from build123d import *

# Parameters (mm, degrees)
SKETCH1_W           = 24
SKETCH1_H           = 6
SKETCH1_H_2         = 24
SKETCH1_W_2         = 6
SKETCH1_R           = 1.625
BOSS_EXTRUDE1_DEPTH = 1.6
FILLET1_R           = 3.5
FILLET2_R           = 5


with BuildPart() as part:
    # Sketch1 → Boss-Extrude1 (new body)
    # profile 1 of 7: a face of its own
    with BuildSketch(Plane(origin=(0, 0, 0), x_dir=(1, 0, 0), z_dir=(0, 1, 0))):
        with Locations((0, 15)):
            Rectangle(SKETCH1_W, SKETCH1_H)
    # profile 2 of 7: a face of its own
    with BuildSketch(Plane(origin=(0, 0, 0), x_dir=(1, 0, 0), z_dir=(0, 1, 0))):
        Rectangle(SKETCH1_W, SKETCH1_H_2)
    # profile 3 of 7: a face of its own
    with BuildSketch(Plane(origin=(0, 0, 0), x_dir=(1, 0, 0), z_dir=(0, 1, 0))):
        with Locations((15, -15)):
            Rectangle(SKETCH1_W_2, SKETCH1_H)
        with Locations(Location((15.25, -15.25, 0), (0, 0, 270))):
            Circle(SKETCH1_R, mode=Mode.SUBTRACT)
    # profile 4 of 7: a face of its own
    with BuildSketch(Plane(origin=(0, 0, 0), x_dir=(1, 0, 0), z_dir=(0, 1, 0))):
        with Locations((0, -15)):
            Rectangle(SKETCH1_W, SKETCH1_H)
    # profile 5 of 7: a face of its own
    with BuildSketch(Plane(origin=(0, 0, 0), x_dir=(1, 0, 0), z_dir=(0, 1, 0))):
        with Locations((-15, -15)):
            Rectangle(SKETCH1_W_2, SKETCH1_H)
        with Locations(Location((-15.25, -15.25, 0), (0, 0, 270))):
            Circle(SKETCH1_R, mode=Mode.SUBTRACT)
    # profile 6 of 7: a face of its own
    with BuildSketch(Plane(origin=(0, 0, 0), x_dir=(1, 0, 0), z_dir=(0, 1, 0))):
        with Locations((15, 15)):
            Rectangle(SKETCH1_W_2, SKETCH1_H)
        with Locations(Location((15.25, 15.25, 0), (0, 0, 270))):
            Circle(SKETCH1_R, mode=Mode.SUBTRACT)
    # profile 7 of 7: a face of its own
    with BuildSketch(Plane(origin=(0, 0, 0), x_dir=(1, 0, 0), z_dir=(0, 1, 0))):
        with Locations((-15, 15)):
            Rectangle(SKETCH1_W_2, SKETCH1_H)
        with Locations(Location((-15.25, 15.25, 0), (0, 0, 270))):
            Circle(SKETCH1_R, mode=Mode.SUBTRACT)
    extrude(amount=BOSS_EXTRUDE1_DEPTH)

    # Fillet1
    # the kernel refuses this fillet: 3.5 mm, written as the material it takes off along each edge
    with BuildSketch(Plane(origin=(-18, -8.75, 12), x_dir=(1, 0, 0), z_dir=(0, 1, 0)), Plane(origin=(-18, -8.75, -12), x_dir=(0, 0, -1), z_dir=(0, 1, 0)), Plane(origin=(18, -8.75, -12), x_dir=(-1, 0, 0), z_dir=(0, 1, 0)), Plane(origin=(18, -8.75, 12), x_dir=(0, 0, 1), z_dir=(0, 1, 0)), Plane(origin=(18, -8.75, 18), x_dir=(-1, 0, 0), z_dir=(0, 1, 0)), Plane(origin=(-18, -8.75, 18), x_dir=(0, 0, -1), z_dir=(0, 1, 0)), Plane(origin=(-18, -8.75, -18), x_dir=(1, 0, 0), z_dir=(0, 1, 0))) as fillet1_piece_1:
        with BuildLine():
            CenterArc((FILLET1_R, -FILLET1_R), FILLET1_R, 90, 90)
            Line((0, -FILLET1_R), (0, 0))
            Line((0, 0), (FILLET1_R, 0))
        make_face()
    extrude(amount=19.1, mode=Mode.SUBTRACT)
    with BuildSketch(Plane(origin=(18, -8.75, -18), x_dir=(-1, 0, 0), z_dir=(0, 1, 0))) as fillet1_piece_2:
        with BuildLine():
            CenterArc((FILLET1_R, FILLET1_R), FILLET1_R, 180, 90)
            Line((0, FILLET1_R), (0, 0))
            Line((0, 0), (FILLET1_R, 0))
        make_face()
    extrude(amount=19.1, mode=Mode.SUBTRACT)

    # Fillet2
    fillet2_edges = [part.edges().sort_by_distance(p)[0] for p in [
        (12, 0.8, -12),
        (12, 0.8, 12),
        (-12, 0.8, 12),
        (-12, 0.8, -12),
    ]]
    fillet(fillet2_edges, radius=FILLET2_R)


solid = part.part
Check sheet for the modelled part. Datum: model origin and axes. Units: mm. A direction names the side the tool comes from. Round coordinates to 2 decimals unless told otherwise and drop trailing zeros. Order: outer loops, then holes, each group sorted by start corner. A loop starts at its lowest first (then second) coordinate and runs counter-clockwise, first axis right, second up.
Q1. Scan lines: L1, parallel to X at y = 1, z = 15.25 (3 decimals); L2, parallel to X at y = 0.85, z = -16; L3, parallel to Z at x = 14, y = 1.2. Record each from-to range of solid material in increasing order.
Filled sheet:
L1: x = -17.919 to -16.875, -13.625 to 13.625, 16.875 to 17.919
L2: x = -17.66 to -16.69, -13.81 to 13.81, 16.69 to 17.66
L3: z = -18 to -16.29, -14.21 to -11.38, 11.38 to 14.21, 16.29 to 18
Q2. Depth check by flat-ended pin: P1, Ø4, axis at x = 15.25, z = 15.25, coming from the -Y side; P2, Ø0.8, axis at y = 0.5, z = 0, coming from the +X side; P3, Ø0.8, axis at y = 0.5, z = 0, coming from the -X side. Enter the tip coordinate at first touch or a pass-through.
Filled sheet:
P1: stops at y = 0
P2: stops at x = 12
P3: stops at x = -12
Q3. Set-up check for faces 5 (the face through (-12, 1, 0)), 6 (the face through (-16.69, 0.79, 16)), 7 (the face through (17.18, 0.79, 13.25)): record each of +Z, -Z, +X, -X, +Y, -Y from which the full face is reachable in a straight line by a thin tool's end or side.
Filled sheet:
face 5: -X, +Y, -Y
face 6: +Y, -Y
face 7: +X, +Y, -Y
Q4. Cross-section at B-B, the plane z = -3.5. Enter the section's corners in (x, y).
Filled sheet:
outline: (-12, 0) - (12, 0) - (12, 1.6) - (-12, 1.6) - close
Q5. Cross-section at A-A, the plane y = 0.95. Give the number of separate pieces and of enclosed holes in the cut face, plus the area to 3 significant figures.
Filled sheet:
separate pieces: 1
enclosed holes: 4
area: 970 mm2
Q6. Draft check along Z on faces 1 (the face through (16.82, 0.79, -17.12)), 2 (the face through (16.76, 0.79, 17.17)), 3 (the face through (13.81, 0.79, -14.5)), 4 (the face through (0, 1.6, 0)). Enter one of: pulls with the +Z half, pulls with the -Z half, needs draft (parallel to the pull), parting line crosses it, or undercut.
Filled sheet:
face 1: pulls with the -Z half
face 2: pulls with the +Z half
face 3: undercut
face 4: needs draft
